from build123d import *

# Parameters (mm, degrees)
F0_W     = 3.2
F0_H     = 90
F0_W_2   = 90
F0_H_2   = 3.2
F1_DEPTH = 1
F2_DEPTH = 4
F3_DEPTH = 100


with BuildPart() as f1:
    # F0 (on Top) → F1 (new body)
    with BuildSketch(Plane.XY):
        with Locations((-34.457693, 13.804672)):
            Rectangle(F0_W, F0_H)
        Polygon((-32.857693, -31.195328), (-36.057693, -31.195328), (-36.057693, -41.195328), (-26.057693, -41.195328), (-26.057693, -37.995328), (-32.857693, -37.995328), align=None)
        Polygon((-26.057693, 58.804672), (-32.857693, 58.804672), (-32.857693, -31.195328), (-26.057693, -37.995328), (63.942307, -37.995328), (63.942307, -31.195328), (-26.057693, -31.195328), align=None)
        with Locations((18.942307, -39.595328)):
            Rectangle(F0_W_2, F0_H_2)
        Polygon((-26.057693, -37.995328), (-32.857693, -31.195328), (-32.857693, -37.995328), align=None)
    extrude(amount=-F1_DEPTH)

    # F0 (on Top) → F2 (join)
    with BuildSketch(Plane.XY):
        with Locations((-34.457693, 13.804672)):
            Rectangle(F0_W, F0_H)
        Polygon((-32.857693, -31.195328), (-36.057693, -31.195328), (-36.057693, -41.195328), (-26.057693, -41.195328), (-26.057693, -37.995328), (-32.857693, -37.995328), align=None)
        with Locations((18.942307, -39.595328)):
            Rectangle(F0_W_2, F0_H_2)
    extrude(amount=F2_DEPTH)

    # F0 (on Top) → F3 (join)
    with BuildSketch(Plane.XY):
        Polygon((-32.857693, -31.195328), (-36.057693, -31.195328), (-36.057693, -41.195328), (-26.057693, -41.195328), (-26.057693, -37.995328), (-32.857693, -37.995328), align=None)
    extrude(amount=F3_DEPTH)


solid = f1.part
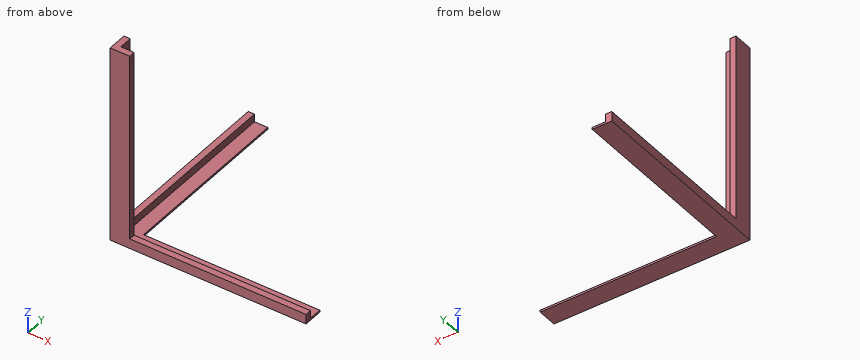
Here's how the part is built. I have some questions about the finished solid (model axes, mm). Round coordinates to 2 decimals unless told otherwise and drop trailing zeros. Order: outer loops, then holes, each group sorted by start corner. A loop starts at its lowest first (then second) coordinate and runs counter-clockwise, first axis right, second up. Notation, with made-up numbers: (-39.5, 39.25) -> (-27.5, 39.25) arc R15 ccw to (-27.5, 59.25) -> close; hole circle Ø4 at (5.25, 55). An arc over 180 degrees is marked (long way). Return JSON: item names as keys, results as strings.
Q1. If we section it at B-B on x = -10.5: List the corners of the cut face in (y, z) for me.
Filled sheet:
{"outline": "(-41.2, -1) -> (-31.2, -1) -> (-31.2, 0) -> (-38, 0) -> (-38, 4) -> (-41.2, 4) -> close"}
Q2. If we section it at A-A on y = -20: List the corners of the cut face in (x, z) for me, plus the area to 3 significant figures.
Filled sheet:
{"outline": "(-36.06, -1) -> (-26.06, -1) -> (-26.06, 0) -> (-32.86, 0) -> (-32.86, 4) -> (-36.06, 4) -> close", "area": "22.8 mm^2"}
Q3. For pin 1 Ø3.5 at (y, z) = (-40.5, 63) entering from +X; pin 2 Ø1.1 at (x, z) = (19.5, -0.5) entering from +Y; pin 3 Ø1 at (x, y) = (38.5, -40) entering from +Z, each with a flat end and sliding along its axis, tell me the tip position at first contact or that it passes through.
Filled sheet:
{"pin 1": "stops at x = -26.06", "pin 2": "stops at y = -31.2", "pin 3": "stops at z = 4"}
Q4. I need wall thicknesses on line 1 along Z through (x, y) = (40, -32); line 2 along Y through (x, z) = (-31, 45). Which ranges of each line are inside material? Lowest first, please. Write a range as from..to.
Filled sheet:
{"line 1": "z = -1..0", "line 2": "y = -41.2..-38"}
